Build history of the part. All positions in model axes, mm. Face numbers are marked on the shaded views. A direction names the side the tool comes from. Round coordinates to 2 decimals unless told otherwise and drop trailing zeros. Write each loop counter-clockwise with the first axis right and the second up, starting at its lowest first coordinate (ties: lowest second). Pieces come first, ordered by that corner, then holes. Notation, with made-up numbers: M -28.5,-17 L -13.5,-17 A23 ccw -13.5,4 Z; hole C -29,-28.75 d1. An arc over 180 degrees is marked long. One line per item, written item: value. Start each with the question number.
```python
from build123d import *

# Parameters (mm, degrees)
F0_R     = 3.175
F0_R_2   = 12.7
F1_DEPTH = 19.05
F2_R     = 25.4
F3_R     = 5.08
F4_R     = 19.05
F4_R_2   = 12.7
F5_DEPTH = 25.4
F6_R     = 2.54


with BuildPart() as f1:
    # F0 (on Front) → F1 (new body)
    with BuildSketch(Plane.XZ):
        with BuildLine():
            ThreePointArc((12.1355523508, -36.115625), (38.1, 0), (12.1355523508, 36.115625))
            ThreePointArc((12.1355523508, 36.115625), (0, 69.85), (-12.1355523508, 36.115625))
            ThreePointArc((-12.1355523508, 36.115625), (-38.1, 0), (-12.1355523508, -36.115625))
            ThreePointArc((-12.1355523508, -36.115625), (0, -69.85), (12.1355523508, -36.115625))
        make_face()
        with Locations((0, -50.8)):
            Circle(F0_R, mode=Mode.SUBTRACT)
        Circle(F0_R_2, mode=Mode.SUBTRACT)
        with Locations((0, 50.8)):
            Circle(F0_R, mode=Mode.SUBTRACT)
    extrude(amount=F1_DEPTH)

    # F2
    f2_edges = [f1.edges().sort_by_distance(p)[0] for p in [
        (12.135552, -9.525, 36.115625),
        (12.135552, -9.525, -36.115625),
        (-12.135552, -9.525, -36.115625),
        (-12.135552, -9.525, 36.115625),
    ]]
    fillet(f2_edges, radius=F2_R)

    # F3
    f3_edges = [f1.edges().sort_by_distance(p)[0] for p in [
        (-20.227695, -19.05, 37.102211),
    ]]
    fillet(f3_edges, radius=F3_R)

    # F4 (on face) → F5 (join)
    with BuildSketch(Plane.XZ.offset(19.05)):
        Circle(F4_R)
        Circle(F4_R_2, mode=Mode.SUBTRACT)
    extrude(amount=F5_DEPTH)

    # F6
    f6_edges = [f1.edges().sort_by_distance(p)[0] for p in [
        (-19.05, -44.45, 0),
    ]]
    fillet(f6_edges, radius=F6_R)


solid = f1.part
```
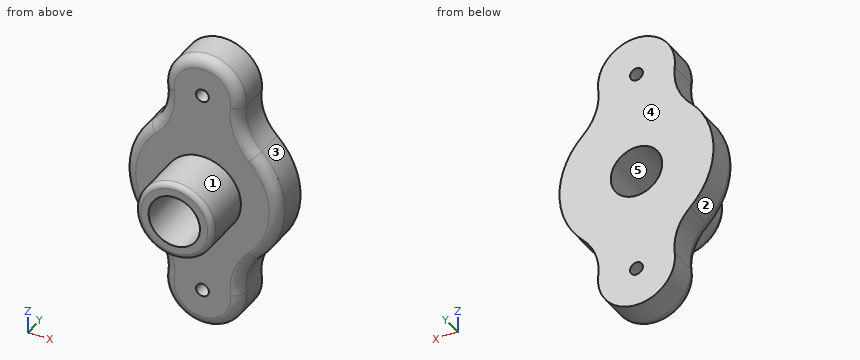
Item 1: Which spindle directions (+Z, -Z, +X, -X, +Y, -Y) get a long thin tool onto all of the face, cutting with end or side? Do the marked faces 1 and 2. Say none if no direction does.
Item 2: Cut at D-D, the plane y = -16. Count the separate pieces of the cut face and the enclosed holes in it, plus the area to 3 significant figures.
Item 3: Cut at B-B, the plane x = 0. Write the cut outline in (y, z) (3 decimals), plus the area to 3 significant figures.
Item 4: Cut at A-A, the plane z = 0. Write the cut outline in (x, y).
Item 5: Two-plate mould, pull along X, no slides. Class the marked faces 3, 4 and 5: pulls with the +X half, pulls with the -X half, needs draft (parallel to the pull), parting line crosses it, or undercut.
Item 6: Drop flat-ended pins along their axis: pin 1 (3 mm diameter, centred on y = -8.5, z = -44.5, fed in from -X); pin 2 (1.5 mm diameter, centred on x = -11, y = -37, fed in from +Z); pin 3 (4 mm diameter, centred on x = -5.5, z = 18, fed in from -Y). Give the stop position or say it passes through.
Item 7: Cut at C-C, the plane y = -29. Write the cut outline in (x, z).
Item 8: Drill centre lines: line 1 (Z direction, x = 0, y = -11) (3 decimals); line 2 (X direction, y = -13, z = 51); line 3 (Y direction, x = -20, z = 4). Where is each one in solid material? Low to high.
Computed values:
1. face 1: -Y
1. face 2: -X, +Y, -Y
2. separate pieces: 1
2. enclosed holes: 3
2. area: 6,140 mm2
3. outline: M -44.45,-16.51 A2.54 ccw -41.91,-19.05 L -19.05,-19.05 L -19.05,-47.625 L 0,-47.625 L 0,-12.7 L -44.45,-12.7 Z; M -44.45,12.7 L 0,12.7 L 0,47.625 L -19.05,47.625 L -19.05,19.05 L -41.91,19.05 A2.54 ccw -44.45,16.51 Z; M -19.05,-64.77 A5.08 ccw -13.97,-69.85 L 0,-69.85 L 0,-53.975 L -19.05,-53.975 Z; M -19.05,53.975 L 0,53.975 L 0,69.85 L -13.97,69.85 A5.08 ccw -19.05,64.77 Z
3. area: 2,240 mm2
4. outline: M -38.1,-13.97 A5.08 ccw -33.02,-19.05 L -19.05,-19.05 L -19.05,-41.91 A2.54 ccw -16.51,-44.45 L -12.7,-44.45 L -12.7,0 L -38.1,0 Z; M 12.7,-44.45 L 16.51,-44.45 A2.54 ccw 19.05,-41.91 L 19.05,-19.05 L 33.02,-19.05 A5.08 ccw 38.1,-13.97 L 38.1,0 L 12.7,0 Z
5. face 3: pulls with the +X half
5. face 4: needs draft
5. face 5: undercut
6. pin 1: stops at x = -18.89
6. pin 2: stops at z = 16.06
6. pin 3: stops at y = -44.43
7. outline: C 0,0 d38.1; hole C 0,0 d25.4
8. line 1: z = -69.85 to -53.975, -47.625 to -12.7, 12.7 to 47.625, 53.975 to 69.85
8. line 2: x = -19.05 to -3.17, 3.17 to 19.05
8. line 3: y = -19.05 to 0
